Drawing for the job (mm, zero at the part's lowest x, y, z). A direction names the side the tool comes from. Round coordinates to 2 decimals unless told otherwise and drop trailing zeros. Write each loop counter-clockwise with the first axis right and the second up, starting at its lowest first coordinate (ties: lowest second). Pieces come first, ordered by that corner, then holes.
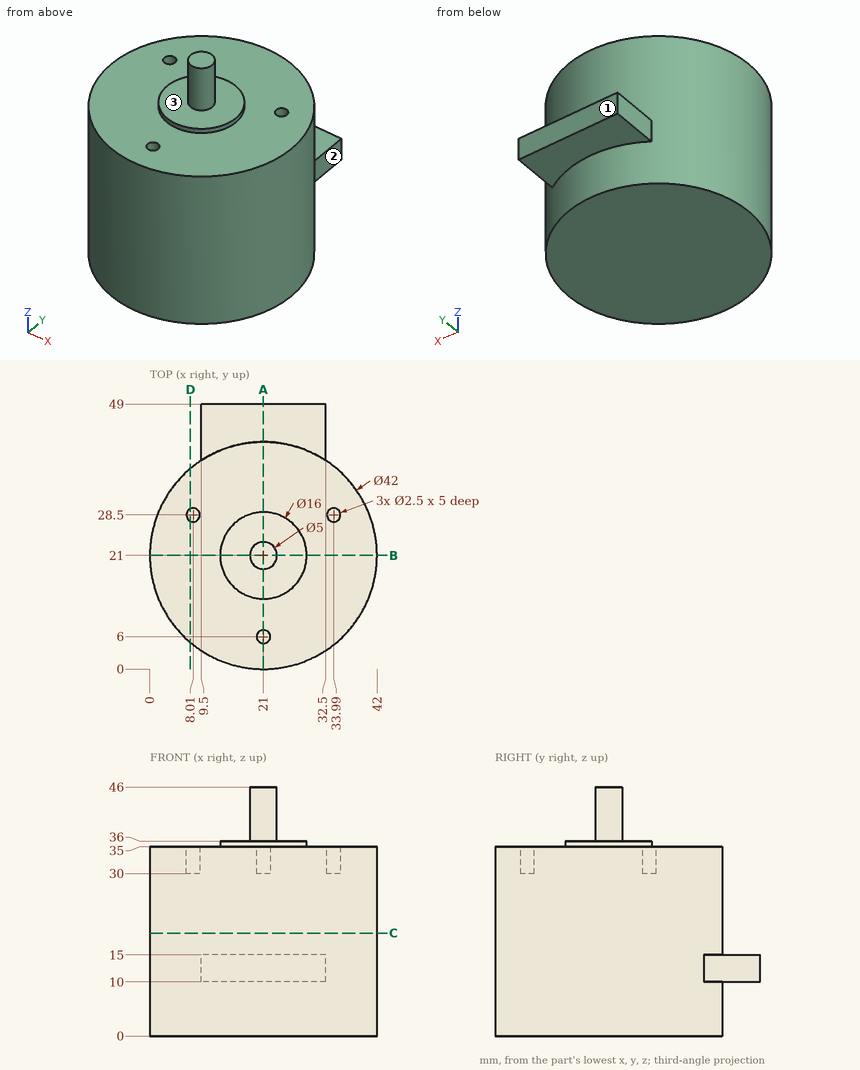
Q1. Drop flat-ended pins along their axis: P1, Ø6, axis at y = 42.5, z = 22, coming from the -X side (1 decimal); P2, Ø1, axis at y = 16.5, z = 12, coming from the -X side (1 decimal); P3, Ø5, axis at x = 37.5, y = 39.5, coming from the -Z side; P4, Ø1, axis at x = 21.5, z = 25, coming from the +Y side. Give the stop position or say it passes through.
Q2. Tool access for the marked faces 1, 2 and 3: list every direction of +Z, -Z, +X, -X, +Y, -Y with a clear straight run to the whole face (end or side of a thin tool).
Q3. Saw through at C-C, the plane z = 19. Write the cut outline in (x, y), and give its area (3 significant figures).
Q4. Saw through at D-D, the plane x = 7.5. Write the cut outline in (y, z) (1 decimal), and give its area (3 significant figures).
Q5. Wall check: line 1 (X direction, y = 28, z = 32) (1 decimal); line 2 (Z direction, x = 25, y = 45); line 3 (Z direction, x = 12.5, y = 14.5). Give the ranges that are in metal, low to high.
Q6. Saw through at A-A, the plane x = 21. Write the cut outline in (y, z).
Q7. Saw through at B-B, the plane y = 21. Write the cut outline in (x, z), and give its area (3 significant figures).
Computed:
1. P1: stops at x = 11.1
1. P2: stops at x = 0.4
1. P3: passes through
1. P4: stops at y = 42
2. face 1: +Z, -Z, +X, -X, +Y
2. face 2: +Z, -Z, +X, +Y
2. face 3: +Z
3. outline: circle Ø42 at (21, 21)
3. area: 1,390 mm2
4. outline: (4.9, 0) - (37.1, 0) - (37.1, 35) - (29.6, 35) - (29.6, 30) - (27.4, 30) - (27.4, 35) - (4.9, 35) - close
4. area: 1,110 mm2
5. line 1: x = 1.2 to 6.9, 9.2 to 32.8, 35.1 to 40.8
5. line 2: z = 10 to 15
5. line 3: z = 0 to 35
6. outline: (0, 0) - (42, 0) - (42, 10) - (49, 10) - (49, 15) - (42, 15) - (42, 35) - (29, 35) - (29, 36) - (23.5, 36) - (23.5, 46) - (18.5, 46) - (18.5, 36) - (13, 36) - (13, 35) - (7.25, 35) - (7.25, 30) - (4.75, 30) - (4.75, 35) - (0, 35) - close
7. outline: (0, 0) - (42, 0) - (42, 35) - (29, 35) - (29, 36) - (23.5, 36) - (23.5, 46) - (18.5, 46) - (18.5, 36) - (13, 36) - (13, 35) - (0, 35) - close
7. area: 1,540 mm2
